Read the model definition and answer for the solid it produces. Units are mm, in the model's axes. A direction names the side the tool comes from. Coordinates: 2 decimals unless noted, no trailing zeros. Order: outer loops, then holes, each group sorted by start corner. A loop starts at its lowest first (then second) coordinate and runs counter-clockwise, first axis right, second up. Notation, with made-up numbers: M -17,2.25 L 32,2.25 A24 ccw 32,33.25 Z; hole C -26.5,-6 d9. An arc over 180 degrees is marked long. Write each question's results on one line, items separated by ' | '.
```python
from build123d import *

# Parameters (mm, degrees)
SKETCH1_R            = 3.4
SKETCH1_W            = 4
SKETCH1_H            = 4
BOSS_EXTRUDE1_DEPTH  = 400
FILLET1_R            = 2.5
FILLET1_OF_MIRROR1_R = 2.5


with BuildPart() as part:
    # Sketch1 → Boss-Extrude1 (new body)
    with BuildSketch(Plane(origin=(0, 0, 0), x_dir=(1, 0, 0), z_dir=(0, 1, 0))):
        Polygon((-4.244365081, 20.8), (4.244365081, 20.8), (8.1, 24.655634919), (8.1, 27.8), (4.1, 27.8), (4.1, 28.9), (5.1, 28.9), (5.1, 30), (13.444365081, 30), (15, 30), (15, 28.444365081), (15, 20.1), (13.9, 20.1), (13.9, 19.1), (12.8, 19.1), (12.8, 23.1), (9.655634919, 23.1), (5.8, 19.244365081), (5.8, 10.755634919), (9.655634919, 6.9), (12.8, 6.9), (12.8, 10.9), (13.9, 10.9), (13.9, 9.9), (15, 9.9), (15, 1.555634919), (15, 0), (13.444365081, 0), (12.8, 0), (12.8, 5.344365081), (8.1, 5.344365081), (4.244365081, 9.2), (-4.244365081, 9.2), (-8.1, 5.344365081), (-12.8, 5.344365081), (-12.8, 0), (-13.444365081, 0), (-15, 0), (-15, 1.555634919), (-15, 9.9), (-13.9, 9.9), (-13.9, 10.9), (-12.8, 10.9), (-12.8, 6.9), (-9.655634919, 6.9), (-5.8, 10.755634919), (-5.8, 19.244365081), (-9.655634919, 23.1), (-12.8, 23.1), (-12.8, 19.1), (-13.9, 19.1), (-13.9, 20.1), (-15, 20.1), (-15, 28.444365081), (-15, 30), (-13.444365081, 30), (-5.1, 30), (-5.1, 28.9), (-4.1, 28.9), (-4.1, 27.8), (-8.1, 27.8), (-8.1, 24.655634919), align=None)
        with Locations(Location((0, 15, 0), (0, 0, 270))):
            Circle(SKETCH1_R, mode=Mode.SUBTRACT)
        with Locations((11.8, 26.8)):
            Rectangle(SKETCH1_W, SKETCH1_H, mode=Mode.SUBTRACT)
        with Locations((-11.8, 26.8)):
            Rectangle(SKETCH1_W, SKETCH1_H, mode=Mode.SUBTRACT)
    boss_extrude1 = extrude(amount=BOSS_EXTRUDE1_DEPTH)

    # Fillet1
    fillet1_edges = [part.edges().sort_by_distance(p)[0] for p in [
        (15, 200, -30),
        (-15, 200, -30),
    ]]
    fillet(fillet1_edges, radius=FILLET1_R)

    # Mirror1: Boss-Extrude1 across plane
    add(boss_extrude1.mirror(Plane.XY))

    # Fillet1 of Mirror1
    fillet1_of_mirror1_edges = [part.edges().sort_by_distance(p)[0] for p in [
        (15, 200, 30),
        (-15, 200, 30),
    ]]
    fillet(fillet1_of_mirror1_edges, radius=FILLET1_OF_MIRROR1_R)


solid = part.part
```
(1) The part is cut by section B-B, the plane x = 0. Write down the section's boundary in (y, z), then the cut area to 3 significant figures.
Conclusion:
outline: M 0,-20.8 L 400,-20.8 L 400,-18.4 L 0,-18.4 Z; M 0,-11.6 L 400,-11.6 L 400,-9.2 L 0,-9.2 Z; M 0,9.2 L 400,9.2 L 400,11.6 L 0,11.6 Z; M 0,18.4 L 400,18.4 L 400,20.8 L 0,20.8 Z | area: 3,840 mm²
(2) Given pin 1 (0.5 mm diameter, centred on y = 200.5, z = -19.5, fed in from +X); pin 2 (0.9 mm diameter, centred on y = 111.5, z = -29, fed in from +X); pin 3 (1 mm diameter, centred on x = 4, y = 350, fed in from +Z); pin 4 (5.5 mm diameter, centred on x = 0, z = 15, fed in from -Y), each flat-ended and moving along its own axis, determine where each tip first touches the part or whether it passes through.
Conclusion:
pin 1: x = 13.9 | pin 2: x = 14.77 | pin 3: z = 28.9 | pin 4: through
(3) Straight lines are drawn through the part: line 1 (Z direction, x = 11.75, y = 174.5); line 2 (X direction, y = 150, z = 25); line 3 (X direction, y = 165, z = 15). For each, find the intervals that lie inside material, in ascending order.
Conclusion:
line 1: -30 to -28.8, -24.8 to -23.1, -6.9 to -5.34, 5.34 to 6.9, 23.1 to 24.8, 28.8 to 30 | line 2: -15 to -13.8, -9.8 to -8.1, 8.1 to 9.8, 13.8 to 15 | line 3: -5.8 to -3.4, 3.4 to 5.8
(4) The part is cut by section A-A, the plane z = 15. Write down the section's boundary in (x, y), then the cut area to 3 significant figures.
Conclusion:
outline: M -5.8,0 L -3.4,0 L -3.4,400 L -5.8,400 Z; M 3.4,0 L 5.8,0 L 5.8,400 L 3.4,400 Z | area: 1,920 mm²
(5) For faces 1 (the flat face through (0, 197, 9.2)), 2 (the flat face through (-9, 197, -30)), determine the directions among +Z, -Z, +X, -X, +Y, -Y from which every point of the face is accessible in a straight line to the end or side of a thin tool.
Conclusion:
face 1: +Y, -Y | face 2: -Z, +X, -X, +Y, -Y
(6) The mould has two halves that part along Z. Classify faces 3 (the flat face through (9, 197, 30)), 4 (the flat face through (9, 197, -30)), 5 (the flat face through (12.8, 197, 0)), 6 (the flat face through (-15, 197, 24)): pulls with the +Z half, pulls with the -Z half, needs draft (parallel to the pull), parting line crosses it, or undercut.
Conclusion:
face 3: pulls with the +Z half | face 4: pulls with the -Z half | face 5: undercut | face 6: needs draft
(7) The part is cut by section C-C, the plane y = 170.5. Count the separate pieces of the cut face and the enclosed holes in it, then the cut area to 3 significant figures.
Conclusion:
separate pieces: 1 | enclosed holes: 7 | area: 577 mm²
